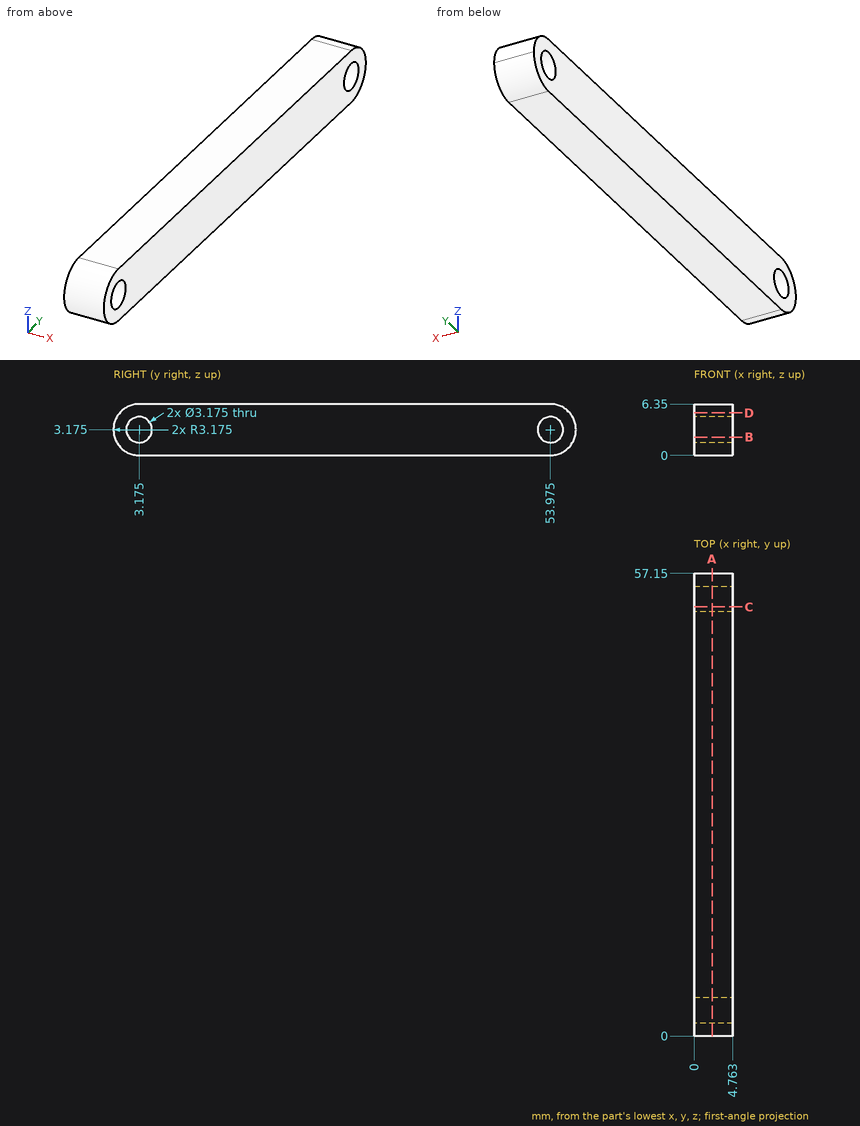
Part print with two shaded views. Sizes in mm from the minimum x, y, z corner. Round coordinates to 2 decimals unless told otherwise and drop trailing zeros. Order: outer loops, then holes, each group sorted by start corner. A loop starts at its lowest first (then second) coordinate and runs counter-clockwise, first axis right, second up. Notation, with made-up numbers: M 47,-25 L 62,-25 A38 cw 62,14 Z; hole C 6,5 d3. An arc over 180 degrees is marked long. Put each result on its own line as item: value. Start each with the question number.
1. Slice it at D-D on z = 5.25. List the corners of the cut face in (x, y), then the cut area to 3 significant figures.
2. Slice it at C-C on y = 53. List the corners of the cut face in (x, z).
3. Slice it at A-A on x = 2.25. State how many separate pieces and enclosed holes the cut face has.
4. Slice it at B-B on z = 2.25. List the corners of the cut face in (x, y) (1 decimal), then the cut area to 3 significant figures.
5. Drill centre lines: probe 1 along Y at (x, z) = (0.5, 3.25); probe 2 along Y at (x, z) = (4, 4.5); probe 3 along Z at (x, y) = (2.1, 4). Where is each one in solid material? Low to high. Write a range as [from, to].
Findings:
1. outline: M 0,0.77 L 4.76,0.77 L 4.76,56.38 L 0,56.38 Z
1. area: 265 mm2
2. outline: M 0,0 L 4.76,0 L 4.76,1.92 L 0,1.92 Z; M 0,4.43 L 4.76,4.43 L 4.76,6.35 L 0,6.35 Z
3. separate pieces: 1
3. enclosed holes: 2
4. outline: M 0,0.1 L 4.8,0.1 L 4.8,1.9 L 0,1.9 Z; M 0,4.5 L 4.8,4.5 L 4.8,52.7 L 0,52.7 Z; M 0,55.3 L 4.8,55.3 L 4.8,57 L 0,57 Z
4. area: 246 mm2
5. probe 1: [0, 1.59], [4.76, 52.39], [55.56, 57.15]
5. probe 2: [0.29, 2.3], [4.05, 53.1], [54.85, 56.86]
5. probe 3: [0, 1.82], [4.53, 6.35]
